The listing builds one solid part. Answer for the finished solid, in the listing's coordinates (mm). Face numbers are marked on the shaded views. A direction names the side the tool comes from. Coordinates: 2 decimals unless noted, no trailing zeros. Write each loop counter-clockwise with the first axis right and the second up, starting at its lowest first coordinate (ties: lowest second). Pieces come first, ordered by that corner, then holes.
Autodesk Inventor part; units mm, degrees
ref_plane "YZ Plane" through (0, 0, 0) normal (1, 0, 0) x (0, 1, 0)
ref_plane "XZ Plane" through (0, 0, 0) normal (0, 1, 0) x (-1, 0, 0)
ref_plane "XY Plane" through (0, 0, 0) normal (0, 0, 1) x (1, 0, 0)
sketch "Sketch3" plane through (0, 0, 0) normal (0, 0, 1) x (1, 0, 0)
  line L0 (0, 0) -> (10, 0)
  line L1 (0, 0) -> (0, 20)
  line L2 (0, 20) -> (8, 20)
  line L3 (10, 0) -> (10, 5)
  line L4 (10, 5) -> (8, 5)
  line L5 (8, 5) -> (8, 7)
  line L6 (8, 7) -> (10, 9.3965)
  line L7 (10, 9.3965) -> (10, 13.3965)
  line L8 (10, 13.3965) -> (8, 20)
  dimension "d17" = 10
  dimension "d18" = 20
  dimension "d19" = 8
  dimension "d40" = 5
  dimension "d43" = 2
  dimension "d44" = 4
  dimension "d45" = 2
revolve "Revolution1" add sketch "Sketch3" angle 360 about axis through (0, 0, 0) along (0, 1, 0)
sketch "Sketch4" plane through (0, 0, 0) normal (0, 1, 0) x (-1, 0, 0)
  circle A0 centre (0, 0) radius 1.5
  dimension "d27" = 3
extrude "Extrusion3" cut sketch "Sketch4" along normal through all
sketch "Sketch5" plane through (0, 20, 0) normal (0, 1, 0) x (1, 0, 0)
  circle A0 centre (0, 0) radius 2.65
  dimension "d30" = 5.3
extrude "Extrusion4" cut sketch "Sketch5" against normal blind 5
sketch "Sketch6" plane through (0, 0, 0) normal (0, -1, 0) x (1, 0, 0)
  circle A0 centre (-6, 0) radius 1.5
  circle A1 centre (6, 0) radius 1.5
  circle A2 centre (0, 0) radius 1.5
  line L0 (-6, 0) -> (0, 0) construction
  line L1 (0, 0) -> (6, 0) construction
  dimension "d33" = 3
  dimension "d35" = 3
  dimension "d47" = 6
extrude "Extrusion5" [suppressed]
equation "\"d35\" = d33"
equation "\"d47\" = 2 * d33"
properties part number "modular-post"
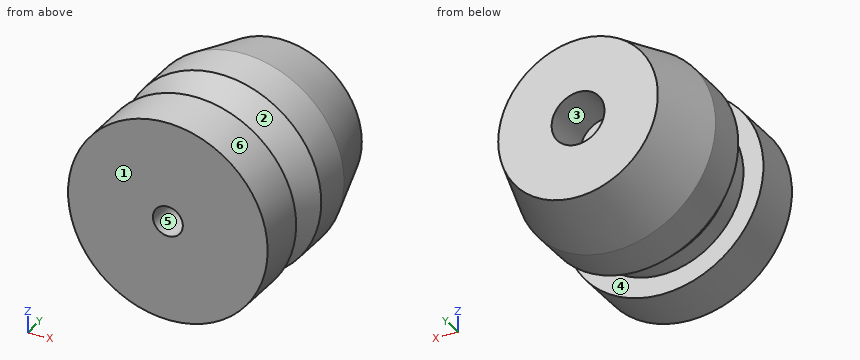
Q1. Determine the mould class of the marked faces 3, 4, 5 and 6 for opening direction Z: released by +Z, released by -Z, zero draft, split by the parting line, or undercut.
Answers below:
face 3: undercut
face 4: zero draft
face 5: undercut
face 6: split by the parting line
Q2. The part is cut by section C-C, the plane y = 11.75. Write down the section's boundary in (x, z), then the cut area to 3 significant figures.
Answers below:
outline: circle Ø20 at (0, 0); hole circle Ø3 at (0, 0)
area: 307 mm2
Q3. The part is cut by section D-D, the plane y = 9. Write down the section's boundary in (x, z).
Answers below:
outline: circle Ø19.34 at (0, 0); hole circle Ø3 at (0, 0)
Q4. Find the intervals of material crossed by probe 1 along X at (y, z) = (9.5, 0); probe 2 along Z at (x, y) = (0, 17.9); probe 3 along X at (y, z) = (17.5, -0.5), in increasing order.
Answers below:
probe 1: x = -10 to -1.5, 1.5 to 10
probe 2: z = -8.64 to -2.65, 2.65 to 8.64
probe 3: x = -8.74 to -2.6, 2.6 to 8.74
Q5. The part is cut by section A-A, the plane x = 0. Write down the section's boundary in (y, z).
Answers below:
outline: (0, -10) - (5, -10) - (5, -8) - (7, -8) - (9.4, -10) - (13.4, -10) - (20, -8) - (20, -2.65) - (15, -2.65) - (15, -1.5) - (0, -1.5) - close; (0, 1.5) - (15, 1.5) - (15, 2.65) - (20, 2.65) - (20, 8) - (13.4, 10) - (9.4, 10) - (7, 8) - (5, 8) - (5, 10) - (0, 10) - close
Q6. The part is cut by section B-B, the plane z = 0. Write down the section's boundary in (x, y).
Answers below:
outline: (-10, 0) - (-1.5, 0) - (-1.5, 15) - (-2.65, 15) - (-2.65, 20) - (-8, 20) - (-10, 13.4) - (-10, 9.4) - (-8, 7) - (-8, 5) - (-10, 5) - close; (1.5, 0) - (10, 0) - (10, 5) - (8, 5) - (8, 7) - (10, 9.4) - (10, 13.4) - (8, 20) - (2.65, 20) - (2.65, 15) - (1.5, 15) - close
Q7. Which of the six approach directions +Z, -Z, +X, -X, +Y, -Y give full straight-line access (tool end or side, diameter ignored) to the marked faces 1 and 2?
Answers below:
face 1: +Z, -Z, +X, -X, -Y
face 2: none
Q8. Given pin 1 (6 mm diameter, centred on x = 5.5, z = -8, fed in from +Y); pin 2 (4 mm diameter, centred on x = 7, y = 8, fed in from -Z); pin 3 (6 mm diameter, centred on x = 4.5, y = 9, fed in from -Z); pin 4 (8 mm diameter, centred on y = 10.5, z = -5, fed in from -X), each flat-ended and moving along its own axis, determine where each tip first touches the part or whether it passes through.
Answers below:
pin 1: stops at y = 20
pin 2: stops at z = -8.31
pin 3: stops at z = -9.88
pin 4: stops at x = -9.95
